```python
from build123d import *

# Parameters (mm, degrees)
F1_DEPTH = 10
F2_R     = 2.4
F3_DEPTH = 2.9972
F7_R     = 5.08
F8_R     = 1.27


# Not quite as in the source:
# - a pattern or mirror of a feature is missing from the dataset's text; its kind, count and spacing are read off the source's solid


with BuildPart() as f1:
    # F0 (on Front) → F1 (new body)
    with BuildSketch(Plane.XZ):
        with BuildLine():
            ThreePointArc((0, 3.9243), (2.7748991414, 2.7748991414), (3.9243, 0))
            Line((3.9243, 0), (3.9243, -2.54))
            Line((3.9243, -2.54), (18.9063833089, -2.54))
            Line((18.9063833089, -2.54), (18.9063833089, 0.4572))
            Line((18.9063833089, 0.4572), (6.9063833089, 0.4572))
            ThreePointArc((6.9063833089, 0.4572), (4.894239586, 4.894239586), (0.4572, 6.9063833089))
            Line((0.4572, 6.9063833089), (0.4572, 18.9063833089))
            Line((0.4572, 18.9063833089), (-2.54, 18.9063833089))
            Line((-2.54, 18.9063833089), (-2.54, 3.9243))
            Line((-2.54, 3.9243), (0, 3.9243))
        make_face()
    extrude(amount=F1_DEPTH)

    # F2 (on face) → F3 (cut, through all)
    with BuildSketch(Plane.XY.offset(0.4572)):
        with Locations((12.9063833089, -5)):
            Circle(F2_R)
    f3 = extrude(amount=-F3_DEPTH, mode=Mode.SUBTRACT)

    # F3_copies: F3 across plane
    add(f3.mirror(Plane(origin=(0, 0, 0), x_dir=(-0.7071067812, 0, -0.7071067812), z_dir=(-0.7071067812, 0, 0.7071067812))), mode=Mode.SUBTRACT)

    # F7
    f7_edges = [f1.edges().sort_by_distance(p)[0] for p in [
        (-2.54, -5, 3.9243),
        (3.9243, -5, -2.54),
    ]]
    fillet(f7_edges, radius=F7_R)

    # F8
    f8_edges = [f1.edges().sort_by_distance(p)[0] for p in [
        (0.4572, -5, 18.906383),
        (0.4572, -5, 6.906383),
        (6.906383, -5, 0.4572),
        (18.906383, -5, 0.4572),
    ]]
    fillet(f8_edges, radius=F8_R)


solid = f1.part
```
Source: CAD feature listing. Evaluate the final solid. Frame: model axes, mm. A direction names the side the tool comes from. Coordinates: 2 decimals unless noted, no trailing zeros. Loops run counter-clockwise (first coordinate to the right, second up) from the corner with the lowest first, then second, coordinate; pieces in that order, holes last. Notation, with made-up numbers: M 89,7 L 114,7 A18 cw 114,28 Z; hole C -8,-24.75 d1. An arc over 180 degrees is marked long. Put each result on its own line as item: value. Start each with the question number.
1) Contact query for flat-ended pins moving along their axis: pin 1 Ø4.5 at (x, y) = (12.91, -5) entering from +Z; pin 2 Ø1.5 at (y, z) = (-1, 8.5) entering from +X; pin 3 Ø12 at (x, z) = (0.5, 7.5) entering from +Y. Output: stop coordinate, or through.
2) Reachability of faces 4 (the face through (11.8, -2.7, 0.457)), 5 (the face through (5, -10, 4)) from +Z, -Z, +X, -X, +Y, -Y: full face, straight path, thin tool, end or side. Return the list, or none.
3) Cut plane D-D on z = 9.5. Return the cut outline in (x, y), then the cut area to 3 significant figures.
4) Cut plane C-C on y = -5. Give the number of separate pieces and of enclosed holes in the cut face, then the cut area to 3 significant figures.
5) Cut plane B-B on z = 12. Return the cut outline in (x, y), then the cut area to 3 significant figures.
6) Cut plane A-A on x = 11.5. Return the cut outline in (y, z), then the cut area to 3 significant figures.
7) Ray query, L1, parallel to X at y = -8.75, z = 16; L2, parallel to X at y = -4.5, z = 0.25. Return the intervals inside material, ascending. Write a range as from..to.
8) Pull-direction query (Y, two-part tool) for faces 1 (the face through (5, 0, 4)), 2 (the face through (10.51, -4.89, -1.02)), 3 (the face through (16, -5, -2.54)); classes: pulls with the +Y half, pulls with the -Y half, needs draft (parallel to the pull), parting line crosses it, or undercut.
The answers:
1. pin 1: passes through
1. pin 2: stops at x = 0.48
1. pin 3: stops at y = 0
2. face 4: +Z, +X, +Y, -Y
2. face 5: +Z, -Z, +X, -X, -Y
3. outline: M -2.54,-10 L 0.46,-10 L 0.46,0 L -2.54,0 Z
3. area: 30.0 mm²
4. separate pieces: 3
4. enclosed holes: 0
4. area: 75.3 mm²
5. outline: M -2.54,-10 L 0.46,-10 L 0.46,-7.22 L -2.54,-7.22 Z; M -2.54,-2.78 L 0.46,-2.78 L 0.46,0 L -2.54,0 Z
5. area: 16.7 mm²
6. outline: M -10,-2.54 L -6.94,-2.54 L -6.94,0.46 L -10,0.46 Z; M -3.06,-2.54 L 0,-2.54 L 0,0.46 L -3.06,0.46 Z
6. area: 18.3 mm²
7. L1: x = -2.54..0.46
7. L2: x = 4.1..10.56, 15.25..18.33
8. face 1: pulls with the +Y half
8. face 2: undercut
8. face 3: needs draft
